Autodesk Fusion 360 part; units mm, degrees
sketch "Sketch1" plane through (0, 0, 0) normal (0, 0, 1) x (1, 0, 0)
  line L0 (0, 0) -> (50, 0)
  line L1 (50, 0) -> (50, 137)
  line L2 (50, 137) -> (0, 137)
  line L3 (0, 137) -> (0, 0)
  line L4 (6, 57.4) -> (11, 57.4)
  line L5 (11, 57.4) -> (11, 55.4)
  line L6 (11, 55.4) -> (6, 55.4)
  line L7 (6, 55.4) -> (6, 57.4)
  line L8 (6, 45.7) -> (11, 45.7)
  line L9 (11, 45.7) -> (11, 43.7)
  line L10 (11, 43.7) -> (6, 43.7)
  line L11 (6, 43.7) -> (6, 45.7)
  line L12 (6, 34) -> (11, 34)
  line L13 (11, 34) -> (11, 32)
  line L14 (11, 32) -> (6, 32)
  line L15 (6, 32) -> (6, 34)
  line L16 (36, 57.4) -> (46.1, 57.4)
  line L17 (46.1, 57.4) -> (46.1, 32)
  line L18 (46.1, 32) -> (36, 32)
  line L19 (36, 32) -> (36, 57.4)
  line L20 (20.9, 57.4) -> (31, 57.4)
  line L21 (31, 57.4) -> (31, 32)
  line L22 (31, 32) -> (20.9, 32)
  line L23 (20.9, 32) -> (20.9, 57.4)
  line L24 (0.1, 79) -> (7.5, 79)
  line L25 (7.5, 79) -> (7.5, 65)
  line L26 (7.5, 65) -> (0.1, 65)
  line L27 (0.1, 65) -> (0.1, 79)
  line L28 (7.5, 65) -> (7.5, 79)
  line L29 (42.5, 79) -> (49.9, 79)
  line L30 (49.9, 79) -> (49.9, 65)
  line L31 (49.9, 65) -> (42.5, 65)
  line L32 (42.5, 65) -> (42.5, 79)
  line L33 (7.5, 79) -> (14.9, 79)
  line L34 (14.9, 79) -> (14.9, 65)
  line L35 (14.9, 65) -> (7.5, 65)
  line L36 (7.5, 65) -> (7.5, 79)
  line L37 (42.5, 79) -> (35.1, 79)
  line L38 (35.1, 79) -> (35.1, 65)
  line L39 (35.1, 65) -> (42.5, 65)
  line L40 (42.5, 65) -> (42.5, 79)
  line L41 (15.25, 79) -> (17.25, 79)
  line L42 (17.25, 79) -> (17.25, 76)
  line L43 (17.25, 76) -> (15.25, 76)
  line L44 (15.25, 76) -> (15.25, 79)
  line L45 (17.6, 79) -> (25, 79)
  line L46 (25, 79) -> (25, 65)
  line L47 (25, 65) -> (17.6, 65)
  line L48 (17.6, 65) -> (17.6, 79)
  line L49 (25, 79) -> (32.4, 79)
  line L50 (32.4, 79) -> (32.4, 65)
  line L51 (32.4, 65) -> (25, 65)
  line L52 (25, 65) -> (25, 79)
  line L53 (32.75, 78.921) -> (34.75, 78.921)
  line L54 (34.75, 78.921) -> (34.75, 75.921)
  line L55 (34.75, 75.921) -> (32.75, 75.921)
  line L56 (32.75, 75.921) -> (32.75, 78.921)
  line L57 (15.25, 68.4103) -> (17.25, 68.4103)
  line L58 (17.25, 68.4103) -> (17.25, 65.4103)
  line L59 (17.25, 65.4103) -> (15.25, 65.4103)
  line L60 (15.25, 65.4103) -> (15.25, 68.4103)
  line L61 (32.75, 68) -> (34.75, 68)
  line L62 (34.75, 68) -> (34.75, 65)
  line L63 (34.75, 65) -> (32.75, 65)
  line L64 (32.75, 65) -> (32.75, 68)
  line L65 (13.6, 131) -> (21.2, 131)
  line L66 (21.2, 131) -> (21.2, 118.3)
  line L67 (21.2, 118.3) -> (13.6, 118.3)
  line L68 (13.6, 118.3) -> (13.6, 131)
  line L69 (21.2, 131) -> (28.8, 131)
  line L70 (28.8, 131) -> (36.4, 131)
  line L71 (36.4, 131) -> (36.4, 118.3)
  line L72 (36.4, 118.3) -> (28.8, 118.3)
  line L73 (28.8, 118.3) -> (28.8, 131)
  line L74 (21.2, 131) -> (28.8, 131)
  line L75 (28.8, 131) -> (28.8, 118.3)
  line L76 (28.8, 118.3) -> (21.2, 118.3)
  line L77 (21.2, 118.3) -> (21.2, 131)
  circle A0 centre (25, 98.3) radius 13
  line L78 (7, 135) -> (12, 135)
  line L79 (12, 135) -> (12, 133)
  line L80 (12, 133) -> (7, 133)
  line L81 (7, 133) -> (7, 135)
  line L82 (38, 135) -> (43, 135)
  line L83 (43, 135) -> (43, 133)
  line L84 (43, 133) -> (38, 133)
  line L85 (38, 133) -> (38, 135)
  line L86 (5, 9) -> (11, 9)
  line L87 (11, 9) -> (11, 3)
  line L88 (11, 3) -> (5, 3)
  line L89 (5, 3) -> (5, 9)
  line L90 (39, 9) -> (45, 9)
  line L91 (45, 9) -> (45, 3)
  line L92 (45, 3) -> (39, 3)
  line L93 (39, 3) -> (39, 9)
  line L94 (16.33, 9) -> (22.33, 9)
  line L95 (22.33, 9) -> (22.33, 3)
  line L96 (22.33, 3) -> (16.33, 3)
  line L97 (16.33, 3) -> (16.33, 9)
  line L98 (27.66, 9) -> (33.66, 9)
  line L99 (33.66, 9) -> (33.66, 3)
  line L100 (33.66, 3) -> (27.66, 3)
  line L101 (27.66, 3) -> (27.66, 9)
  line L102 (7, 26) -> (13, 26)
  line L103 (13, 26) -> (13, 20)
  line L104 (13, 20) -> (7, 20)
  line L105 (7, 20) -> (7, 26)
  line L106 (7, 17.5) -> (13, 17.5)
  line L107 (13, 17.5) -> (13, 11.5)
  line L108 (13, 11.5) -> (7, 11.5)
  line L109 (7, 11.5) -> (7, 17.5)
  circle A1 centre (4, 116) radius 1.5
  circle A2 centre (46, 116) radius 1.5
  line L110 (0, 137) -> (5, 137)
  line L111 (5, 137) -> (5, 122)
  line L112 (5, 122) -> (0, 122)
  line L113 (0, 122) -> (0, 137)
  line L114 (50, 137) -> (45, 137)
  line L115 (45, 137) -> (45, 122)
  line L116 (45, 122) -> (50, 122)
  line L117 (50, 122) -> (50, 137)
  circle A3 centre (25, 98.3) radius 7.5
  dimension "d1" = 50
  dimension "d2" = 137
  dimension "d4" = 2
  dimension "d5" = 6
  dimension "d6" = 5
  dimension "d7" = 2
  dimension "d8" = 6
  dimension "d9" = 5
  dimension "d10" = 2
  dimension "d11" = 6
  dimension "d16" = 32
  dimension "d17" = 10.1
  dimension "d18" = 25.4
  dimension "d19" = 32
  dimension "d20" = 25.4
  dimension "d21" = 9.7
  dimension "d22" = 10.1
  dimension "d23" = 25.4
  dimension "d24" = 32
  dimension "d25" = 5
  dimension "d26" = 7.4
  dimension "d27" = 14
  dimension "d29" = 65
  dimension "d45" = 0.1
  dimension "d47" = 14
  dimension "d48" = 0.1
  dimension "d50" = 14
  dimension "d52" = 14
  dimension "d53" = 65
  dimension "d56" = 2
  dimension "d57" = 3
  dimension "d58" = 0.35
  dimension "d59" = 7.4
  dimension "d60" = 14
  dimension "d61" = 0.35
  dimension "d62" = 7.4
  dimension "d63" = 14
  dimension "d64" = 2
  dimension "d65" = 3
  dimension "d66" = 0.35
  dimension "d67" = 2
  dimension "d68" = 3
  dimension "d69" = 0.35
  dimension "d70" = 2
  dimension "d71" = 3
  dimension "d72" = 0.35
  dimension "d73" = 7.6
  dimension "d74" = 12.7
  dimension "d75" = 7.6
  dimension "d76" = 7.6
  dimension "d77" = 12.7
  dimension "d78" = 6
  dimension "d79" = 13.6
  dimension "d80" = 26
  dimension "d81" = 25
  dimension "d82" = 20
  dimension "d83" = 5
  dimension "d84" = 2
  dimension "d85" = 5
  dimension "d86" = 2
  dimension "d87" = 7
  dimension "d88" = 7
  dimension "d91" = 6
  dimension "d92" = 6
  dimension "d93" = 5
  dimension "d94" = 6
  dimension "d95" = 6
  dimension "d96" = 3
  dimension "d97" = 3
  dimension "d98" = 5
  dimension "d101" = 6
  dimension "d102" = 6
  dimension "d103" = 5.33
  dimension "d104" = 5.33
  dimension "d105" = 6
  dimension "d106" = 6
  dimension "d107" = 6
  dimension "d108" = 6
  dimension "d109" = 2.5
  dimension "d110" = 2.5
  dimension "d111" = 7
  dimension "d112" = 7
  dimension "d113" = 3
  dimension "d114" = 3
  dimension "d115" = 21
  dimension "d116" = 4
  dimension "d117" = 4
  dimension "d118" = 21
  dimension "d133" = 5
  dimension "d134" = 15
  dimension "d135" = 5
  dimension "d136" = 15
  dimension "d151" = 2
  dimension "d152" = 2
  dimension "d153" = 15
extrude "Extrude3" add sketch "Sketch1" against normal blind 1.6 contours L0 L1 L2 L3 L111 L112 L115 L116 | L2 L3 L110 L111 L112 L113 | L1 L2 L114 L115 L116 L117 | L4 L5 L6 L7 | L8 L9 L10 L11 | L12 L13 L14 L15 | L16 L17 L18 L19 | L20 L21 L22 L23 | L24 L25 L26 L27 L28 L36 | L25 L28 L33 L34 L35 L36 | L29 L30 L31 L32 L40 | L32 L37 L38 L39 L40 | L41 L42 L43 L44 | L45 L46 L47 L48 L52 | L46 L49 L50 L51 L52 | L53 L54 L55 L56 | L57 L58 L59 L60 | L61 L62 L63 L64 | L65 L66 L67 L68 L77 | L66 L69 L73 L74 L75 L76 L77 | L70 L71 L72 L73 L75 | A0 | L78 L79 L80 L81 | L82 L83 L84 L85 | L86 L87 L88 L89 | L90 L91 L92 L93 | L94 L95 L96 L97 | L98 L99 L100 L101 | L102 L103 L104 L105 | L106 L107 L108 L109 | A3
extrude "Extrude4" add sketch "Sketch1" along normal blind 7.2 contours L24 L25 L26 L27 L28 L36 | L25 L28 L33 L34 L35 L36 | L29 L30 L31 L32 L40 | L32 L37 L38 L39 L40 | L45 L46 L47 L48 L52 | L46 L49 L50 L51 L52
extrude "Extrude5" add sketch "Sketch1" along normal blind 7 contours L65 L66 L67 L68 L77 | L66 L69 L73 L74 L75 L76 L77 | L70 L71 L72 L73 L75
extrude "Extrude6" add sketch "Sketch1" along normal blind 7.2 contours L16 L17 L18 L19 | L20 L21 L22 L23
extrude "Extrude7" add sketch "Sketch1" along normal blind 7.2 contours L4 L5 L6 L7 | L8 L9 L10 L11 | L12 L13 L14 L15
extrude "Extrude8" cut sketch "Sketch1" against normal blind 15 contours L2 L3 L110 L111 L112 L113 | L1 L2 L114 L115 L116 L117
extrude "Extrude9" add sketch "Sketch1" along normal blind 7.9 contours A0 | A3
extrude "Extrude10" add 1 faces at (21.0958, 100.1802, 7.9) along direction (0, 0, 1) blind 2
extrude "Extrude11" add 1 faces at (21.0958, 100.1802, 9.9) along direction (0, 0, 1) blind 6
extrude "Extrude12" add 1 faces at (28.8, 122.5333, 7) along direction (0, 0, 1) blind 8
extrude "Extrude13" cut 1 faces at (21.0958, 100.1802, 15.9) along direction (0, 0, -1) blind 10
extrude "Extrude14" cut 1 faces at (28.8, 122.5333, 15) along direction (0, 0, -1) blind 5
extrude "Extrude15" add sketch "Sketch1" along normal blind 5 contours L86 L87 L88 L89 | L90 L91 L92 L93 | L94 L95 L96 L97 | L98 L99 L100 L101 | L102 L103 L104 L105 | L106 L107 L108 L109
Input: part model. Units: mm. Frame: model coordinates. A direction names the side the tool comes from. Give positions to 0.01 mm unless a question says otherwise; leave off trailing zeros. Loops run counter-clockwise (first coordinate to the right, second up) from the corner with the lowest first, then second, coordinate; pieces in that order, holes last. Notation, with made-up numbers: M -7.5,59 L 6.5,59 A15 cw 6.5,80 Z; hole C 80,9.25 d11. An arc over 180 degrees is marked long. Use one line per item in the form item = value.
1. Section query C-C, the plane x = 43. Return the cut outline in (y, z).
Numbers:
outline = M 0,-1.6 L 137,-1.6 L 137,0 L 79,0 L 79,7.2 L 65,7.2 L 65,0 L 57.4,0 L 57.4,7.2 L 32,7.2 L 32,0 L 9,0 L 9,5 L 3,5 L 3,0 L 0,0 Z
2. Line query: L1, parallel to X at y = 116, z = -1.1; L2, parallel to X at y = 70.5, z = 5.5; L3, parallel to Y at x = 46, z = -0.5. Output: solid intervals per line, ascending.
Numbers:
L1 = 0 to 2.5, 5.5 to 44.5, 47.5 to 50
L2 = 0.1 to 14.9, 17.6 to 32.4, 35.1 to 49.9
L3 = 0 to 114.5, 117.5 to 122
3. First-contact query: pin 1 (6 mm diameter, centred on y = 62.5, z = 2, fed in from +X); pin 2 (1.5 mm diameter, centred on x = 20, z = 1.5, fed in from -Y); pin 3 (1.5 mm diameter, centred on x = 10, z = 2.5, fed in from +Y); pin 4 (8 mm diameter, centred on x = 11, y = 94, fed in from +Z). Flat tips, straight axial feed; report the tip coordinate or a pass-through.
Numbers:
pin_1 = 50
pin_2 = 3
pin_3 = 79
pin_4 = 5.9
4. Section query D-D, the plane z = 3.5. Count the separate pieces of the cut face and the enclosed holes in it, and give its area (3 significant figures).
Numbers:
separate_pieces = 16
enclosed_holes = 0
area = 2,200 mm²
5. Section query A-A, the plane y = 116. Return the cut outline in (x, z).
Numbers:
outline = M 0,-1.6 L 2.5,-1.6 L 2.5,0 L 0,0 Z; M 5.5,-1.6 L 44.5,-1.6 L 44.5,0 L 5.5,0 Z; M 47.5,-1.6 L 50,-1.6 L 50,0 L 47.5,0 Z
6. Pull-direction query (X, two-part tool) for faces 5 (the face through (10, 20, 2)), 6 (the face through (27.66, 6, 2)); classes: released by +X, released by -X, zero draft, split by the parting line, or undercut.
Numbers:
face_5 = zero draft
face_6 = undercut
7. Reachability of faces 1 (the face through (31, 45, 4)), 2 (the face through (39, 6, 2)), 3 (the face through (31, 6, 5)), 4 (the face through (25, 79, 4)) from +Z, -Z, +X, -X, +Y, -Y: full face, straight path, thin tool, end or side. Return the list, or none.
Numbers:
face_1 = +Z
face_2 = +Z, -Y
face_3 = +Z, +X, -X, -Y
face_4 = +Z, +X, -X
8. Section query B-B, the plane y = 38.5. Return the cut outline in (x, z).
Numbers:
outline = M 0,-1.6 L 50,-1.6 L 50,0 L 46.1,0 L 46.1,7.2 L 36,7.2 L 36,0 L 31,0 L 31,7.2 L 20.9,7.2 L 20.9,0 L 0,0 Z
